from build123d import *

# Parameters (mm, degrees)
BOSS_EXTRUDE1_DEPTH = 6.35


with BuildPart() as part:
    # Sketch1 → Boss-Extrude1 (new body)
    with BuildSketch(Plane(origin=(0, 0, 0), x_dir=(1, 0, 0), z_dir=(0, 1, 0))):
        with BuildLine():
            ThreePointArc((13.925943024, -1.438092792), (13.981473498, -0.719999187), (14, 0))
            ThreePointArc((14, 0), (11.748311638, 7.614274335), (5.717546621, 12.779266827))
            ThreePointArc((5.717546621, 12.779266827), (0, 10.95), (-5.717546621, 12.779266827))
            ThreePointArc((-5.717546621, 12.779266827), (-12.124355653, 7), (-13.925943024, -1.438092792))
            ThreePointArc((-13.925943024, -1.438092792), (-9.728304381, -5.072629445), (-8.163328399, -10.4))
            ThreePointArc((-8.163328399, -10.4), (-8.174601851, -10.871126227), (-8.208396403, -11.341174035))
            ThreePointArc((-8.208396403, -11.341174035), (0, -14), (8.208396403, -11.341174035))
            ThreePointArc((8.208396403, -11.341174035), (9.482978171, -5.475), (13.925943024, -1.438092792))
        make_face()
    extrude(amount=BOSS_EXTRUDE1_DEPTH)


solid = part.part
Build history of the part. All positions in model axes, mm. Give positions to 0.01 mm unless a question says otherwise; leave off trailing zeros. Order: outer loops, then holes, each group sorted by start corner. A loop starts at its lowest first (then second) coordinate and runs counter-clockwise, first axis right, second up. Notation, with made-up numbers: M -10.5,16 L 9.5,16 A27 ccw 9.5,47 Z; hole C 27.5,0 d8. An arc over 180 degrees is marked long. Use one line per item in the form item = value.
Q1. Pull direction X, two halves, no side cores. Call faces 1 (the cylindrical face through (-12.06, 3.13, -7.11)), 2 (the cylindrical face through (0.09, 3.13, -10.95)), 3 (the flat face through (0, 6.35, 0)): released by +X, released by -X, zero draft, split by the parting line, or undercut.
Conclusion:
face_1 = released by -X
face_2 = undercut
face_3 = zero draft
Q2. Pin check, flat tip, straight feed: P1, Ø1.5, axis at y = 2, z = 2, coming from the -X side. Stop position of the tip, or through.
Conclusion:
P1 = -13.94
Q3. Slice it at B-B, the plane x = 5. Write the cut outline in (y, z).
Conclusion:
outline = M 0,-12.31 L 6.35,-12.31 L 6.35,13.08 L 0,13.08 Z
Q4. Wall check: probe 1 along X at (y, z) = (6, -1.5); probe 2 along X at (y, z) = (2.25, 10.25); probe 3 along Z at (x, y) = (5.75, 1.75). Give the ranges that are in metal, low to high.
Conclusion:
probe_1 = -13.92 to 13.92
probe_2 = -8.16 to 8.16
probe_3 = -12.76 to 12.76
Q5. Slice it at A-A, the plane y = 4.25. Write the cut outline in (x, z).
Conclusion:
outline = M -13.93,1.44 A14 ccw -5.72,-12.78 A9.85 cw 5.72,-12.78 A14 ccw 13.93,1.44 A9.85 cw 8.21,11.34 A14 ccw -8.21,11.34 A9.85 cw Z
Q6. Slice it at C-C, the plane z = 3.75. Write the cut outline in (x, y).
Conclusion:
outline = M -10.75,0 L 10.75,0 L 10.75,6.35 L -10.75,6.35 Z
